Read the model definition and answer for the solid it produces. Units are mm, in the model's axes. Coordinates: 2 decimals unless noted, no trailing zeros. Loops run counter-clockwise (first coordinate to the right, second up) from the corner with the lowest first, then second, coordinate; pieces in that order, holes last. Notation, with made-up numbers: (24, 64) -> (60, 64) arc R25 ccw to (60, 86) -> close; hole circle Ø4 at (-26.75, -34). An arc over 180 degrees is marked (long way). One line per question, with ' | ' between items. Start each with the question number.
```python
from build123d import *

# Parameters (mm, degrees)
BOSS_EXTRUDE1_DEPTH          = 60
M1_6X0_35_TAPPED_HOLE1_D     = 1.25
M1_6X0_35_TAPPED_HOLE1_DEPTH = 2.4
LPATTERN1_COUNT              = 6
LPATTERN1_PITCH              = 10


with BuildPart() as part:
    # Sketch1 → Boss-Extrude1 (new body)
    with BuildSketch(Plane.XY):
        with BuildLine():
            Line((-1.5, 1), (-1.3, 1.2))
            Line((-1.3, 1.2), (1.3, 1.2))
            Line((1.3, 1.2), (1.5, 1))
            Line((1.5, 1), (1.5, 0.8))
            ThreePointArc((1.5, 0.8), (1.3, 0.6), (1.5, 0.4))
            Line((1.5, 0.4), (1.5, -1))
            Line((1.5, -1), (1.3, -1.2))
            Line((1.3, -1.2), (-1.3, -1.2))
            Line((-1.3, -1.2), (-1.5, -1))
            Line((-1.5, -1), (-1.5, 0.4))
            ThreePointArc((-1.5, 0.4), (-1.3, 0.6), (-1.5, 0.8))
            Line((-1.5, 0.8), (-1.5, 1))
        make_face()
    extrude(amount=BOSS_EXTRUDE1_DEPTH)

    # M1.6x0.35 Tapped Hole1
    with Locations(Plane(origin=(0, 1.2, 0), x_dir=(1, 0, 0), z_dir=(0, 1, 0))):
        with Locations((0, -5)):
            m1_6x0_35_tapped_hole1 = Hole(M1_6X0_35_TAPPED_HOLE1_D / 2, depth=M1_6X0_35_TAPPED_HOLE1_DEPTH)

    # LPattern1: M1.6x0.35 Tapped Hole1 ×6
    with Locations(*[(0, 0, i * LPATTERN1_PITCH) for i in range(1, LPATTERN1_COUNT)]):
        add(m1_6x0_35_tapped_hole1, mode=Mode.SUBTRACT)


solid = part.part
```
(1) Section A-A on x = 0 is taken. Write down the section's boundary in (y, z) (3 decimals).
(2) Section D-D on z = 23 is taken. Write down the section's boundary in (x, y), plus the area to 3 significant figures.
(3) Section C-C on y = -0.35 is taken. Write down the section's boundary in (x, z) (3 decimals).
(4) Determine the mould class of faces 1 (the flat face through (0, 1.2, 30)), 2 (the flat face through (-1.5, 0, 30)), 3 (the cylindrical face through (0.08, -0.02, 44.38)) for opening direction X: +X half, -X half, draft (parallel to the pull), parting line (faces both ways), or undercut.
(5) Find the intervals of material crossed by probe 1 along X at (y, z) = (-0.7, 55) (3 decimals); probe 2 along X at (y, z) = (0.55, 26), in increasing order. Write a range as from..to.
(6) Section B-B on z = 15 is taken. Write down the section's boundary in (x, y) (3 decimals), plus the area to 3 significant figures.
Working result:
1) outline: (-1.2, 0) -> (1.2, 0) -> (1.2, 4.375) -> (-1.2, 4.375) -> close; (-1.2, 5.625) -> (1.2, 5.625) -> (1.2, 14.375) -> (-1.2, 14.375) -> close; (-1.2, 15.625) -> (1.2, 15.625) -> (1.2, 24.375) -> (-1.2, 24.375) -> close; (-1.2, 25.625) -> (1.2, 25.625) -> (1.2, 34.375) -> (-1.2, 34.375) -> close; (-1.2, 35.625) -> (1.2, 35.625) -> (1.2, 44.375) -> (-1.2, 44.375) -> close; (-1.2, 45.625) -> (1.2, 45.625) -> (1.2, 54.375) -> (-1.2, 54.375) -> close; (-1.2, 55.625) -> (1.2, 55.625) -> (1.2, 60) -> (-1.2, 60) -> close
2) outline: (-1.5, -1) -> (-1.3, -1.2) -> (1.3, -1.2) -> (1.5, -1) -> (1.5, 0.4) arc R0.2 cw to (1.5, 0.8) -> (1.5, 1) -> (1.3, 1.2) -> (-1.3, 1.2) -> (-1.5, 1) -> (-1.5, 0.8) arc R0.2 cw to (-1.5, 0.4) -> close | area: 6.99 mm2
3) outline: (-1.5, 0) -> (1.5, 0) -> (1.5, 60) -> (-1.5, 60) -> close; hole circle Ø1.25 at (0, 5); hole circle Ø1.25 at (0, 15); hole circle Ø1.25 at (0, 25); hole circle Ø1.25 at (0, 35); hole circle Ø1.25 at (0, 45); hole circle Ø1.25 at (0, 55)
4) face 1: draft | face 2: -X half | face 3: undercut
5) probe 1: x = -1.5..-0.625, 0.625..1.5 | probe 2: x = -1.31..1.31
6) outline: (-1.5, -1) -> (-1.3, -1.2) -> (-0.625, -1.2) -> (-0.625, 1.2) -> (-1.3, 1.2) -> (-1.5, 1) -> (-1.5, 0.8) arc R0.2 cw to (-1.5, 0.4) -> close; (0.625, -1.2) -> (1.3, -1.2) -> (1.5, -1) -> (1.5, 0.4) arc R0.2 cw to (1.5, 0.8) -> (1.5, 1) -> (1.3, 1.2) -> (0.625, 1.2) -> close | area: 3.99 mm2
